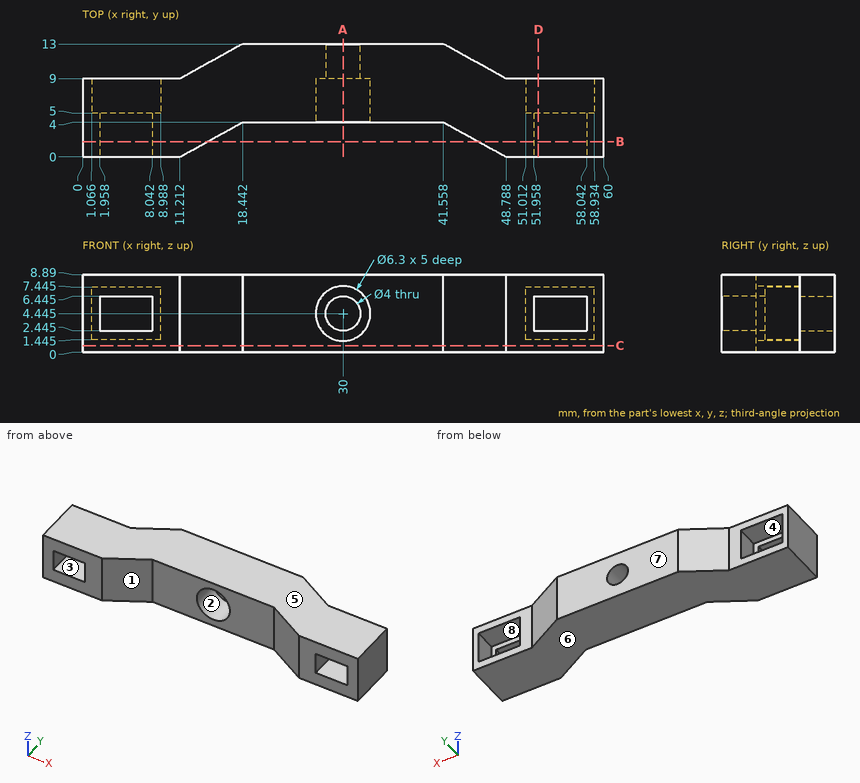
Geometry: see drawing. Coordinates: mm, zero at the bounding-box minimum. A direction names the side the tool comes from. Coordinates: 2 decimals unless noted, no trailing zeros. Loops run counter-clockwise (first coordinate to the right, second up) from the corner with the lowest first, then second, coordinate; pieces in that order, holes last. Notation, with made-up numbers: (45, -22) - (86, -22) arc R16 ccw to (86, 5) - close; hole circle Ø10 at (-31.5, 76.5). An arc over 180 degrees is marked (long way). Answer as CSV lines item,"result".
1. Section C-C (z = 0.75). Return loops of the section in (x, y), then the cut area to 3 significant figures.
Established:
outline,"(0, 0) - (11.21, 0) - (18.44, 4) - (41.56, 4) - (48.79, 0) - (60, 0) - (60, 9) - (48.79, 9) - (41.56, 13) - (18.44, 13) - (11.21, 9) - (0, 9) - close"
area,"540 mm2"
2. Section A-A (x = 30). Return loops of the section in (y, z) (1 decimal).
Established:
outline,"(4, 0) - (13, 0) - (13, 2.4) - (9, 2.4) - (9, 1.3) - (4, 1.3) - close; (4, 7.6) - (9, 7.6) - (9, 6.4) - (13, 6.4) - (13, 8.9) - (4, 8.9) - close"
3. Mould query, pull axis Z, two halves, no side actions, for the marked faces 5, 6, 7 and 8. Classes: released by +Z, released by -Z, zero draft, split by the parting line, or undercut.
Established:
face 5,"released by +Z"
face 6,"released by -Z"
face 7,"zero draft"
face 8,"undercut"
4. Reachability of the marked faces 1, 2, 3 and 4 from +Z, -Z, +X, -X, +Y, -Y: full face, straight path, thin tool, end or side. Return the list, or none.
Established:
face 1,"+Z, -Z, -Y"
face 2,"-Y"
face 3,"+Y, -Y"
face 4,"+Y"
5. Section B-B (y = 1.75). Return loops of the section in (x, z) (1 decimal), then the cut area to 3 significant figures.
Established:
outline,"(0, 0) - (14.4, 0) - (14.4, 8.9) - (0, 8.9) - close; (45.6, 0) - (60, 0) - (60, 8.9) - (45.6, 8.9) - close; hole (2, 2.4) - (8, 2.4) - (8, 6.4) - (2, 6.4) - close; hole (52, 2.4) - (58, 2.4) - (58, 6.4) - (52, 6.4) - close"
area,"207 mm2"
6. Ray query, line 1 (Z direction, x = 30, y = 6.05) (1 decimal); line 2 (Z direction, x = 30, y = 9.95) (1 decimal); line 3 (X direction, y = 2, z = 3.25) (1 decimal). Return the intervals inside material, ascending.
Established:
line 1,"z = 0 to 1.3, 7.6 to 8.9"
line 2,"z = 0 to 2.4, 6.4 to 8.9"
line 3,"x = 0 to 2, 8 to 14.8, 45.2 to 52, 58 to 60"
7. Section D-D (x = 52.5). Return loops of the section in (y, z) (1 decimal).
Established:
outline,"(0, 0) - (9, 0) - (9, 1.4) - (5, 1.4) - (5, 2.4) - (0, 2.4) - close; (0, 6.4) - (5, 6.4) - (5, 7.4) - (9, 7.4) - (9, 8.9) - (0, 8.9) - close"
8. Contact query for flat-ended pins moving along their axis: pin 1 (5 mm diameter, centred on x = 5.5, z = 5, fed in from +Y); pin 2 (3 mm diameter, centred on x = 56, z = 4.5, fed in from +Y); pin 3 (2.5 mm diameter, centred on x = 56, z = 5.5, fed in from +Y); pin 4 (4.5 mm diameter, centred on x = 32.5, z = 3, fed in from -Y). Output: stop coordinate, or through.
Established:
pin 1,"stops at y = 9"
pin 2,"passes through"
pin 3,"stops at y = 5"
pin 4,"stops at y = 4"
